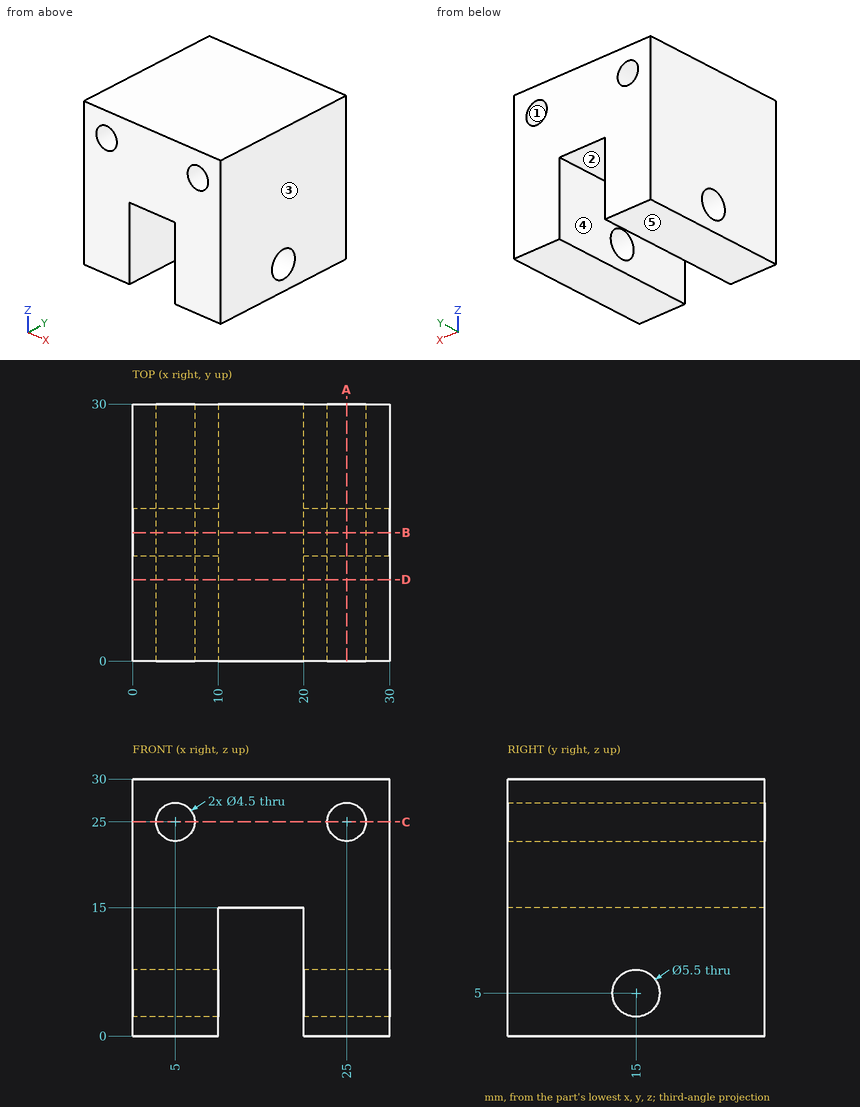
The figure shows three views and two pictorial views of one solid part (mm, origin at its lowest corner). Answer the questions. A direction names the side the tool comes from. Round coordinates to 2 decimals unless told otherwise and drop trailing zeros. Order: outer loops, then holes, each group sorted by start corner. A loop starts at its lowest first (then second) coordinate and runs counter-clockwise, first axis right, second up.
Q1. Find the intervals of material crossed by line 1 along X through (y, z) = (2.75, 5.5); line 2 along Z through (x, y) = (5, 21.5); line 3 along Y through (x, z) = (28, 5), in increasing order.
Solution:
line 1: x = 0 to 10, 20 to 30
line 2: z = 0 to 22.75, 27.25 to 30
line 3: y = 0 to 12.25, 17.75 to 30
Q2. A cutting plane is placed at A-A, the plane x = 25. Determine the outline of the cut face in (y, z), then the cut area to 3 significant figures.
Solution:
outline: (0, 0) - (30, 0) - (30, 22.75) - (0, 22.75) - close; (0, 27.25) - (30, 27.25) - (30, 30) - (0, 30) - close; hole circle Ø5.5 at (15, 5)
area: 741 mm2
Q3. A cutting plane is placed at D-D, the plane y = 9.5. Determine the outline of the cut face in (x, z).
Solution:
outline: (0, 0) - (10, 0) - (10, 15) - (20, 15) - (20, 0) - (30, 0) - (30, 30) - (0, 30) - close; hole circle Ø4.5 at (5, 25); hole circle Ø4.5 at (25, 25)
Q4. A cutting plane is placed at B-B, the plane y = 15. Determine the outline of the cut face in (x, z).
Solution:
outline: (0, 0) - (10, 0) - (10, 2.25) - (0, 2.25) - close; (0, 7.75) - (10, 7.75) - (10, 15) - (20, 15) - (20, 7.75) - (30, 7.75) - (30, 30) - (0, 30) - close; (20, 0) - (30, 0) - (30, 2.25) - (20, 2.25) - close; hole circle Ø4.5 at (5, 25); hole circle Ø4.5 at (25, 25)
Q5. The mould has two halves that part along Z. Classify the marked faces 1, 2 and 3: pulls with the +Z half, pulls with the -Z half, needs draft (parallel to the pull), parting line crosses it, or undercut.
Solution:
face 1: undercut
face 2: pulls with the -Z half
face 3: needs draft
Q6. A cutting plane is placed at C-C, the plane z = 25. Determine the outline of the cut face in (x, y), then the cut area to 3 significant figures.
Solution:
outline: (0, 0) - (2.75, 0) - (2.75, 30) - (0, 30) - close; (7.25, 0) - (22.75, 0) - (22.75, 30) - (7.25, 30) - close; (27.25, 0) - (30, 0) - (30, 30) - (27.25, 30) - close
area: 630 mm2
Q7. Given pin 1 Ø11 at (x, y) = (17, 13) entering from -Z, flat-ended and moving along its own axis, determine where the tip first touches the part or whether it passes through.
Solution:
pin 1: stops at z = 0
Q8. A tool of negligible diameter and unlimited length cuts with its end or side. For the marked faces 4 and 5, from which of +Z, -Z, +X, -X, +Y, -Y can it reach the whole face along a straight path? Write none if from no direction.
Solution:
face 4: -Z, +Y, -Y
face 5: -Z, +X, -X, +Y, -Y
